Input: dimensioned drawing with shaded views. Units: mm. Origin: part minimum x, y, z. A direction names the side the tool comes from. Give positions to 0.01 mm unless a question says otherwise; leave off trailing zeros. Loops run counter-clockwise (first coordinate to the right, second up) from the corner with the lowest first, then second, coordinate; pieces in that order, holes last. Notation, with made-up numbers: (65, 57) -> (73, 57) arc R4 cw to (73, 62) -> close; hole circle Ø8 at (82.5, -27). An arc over 180 degrees is marked (long way). One line per question, with ' | ' between items. Start each with the question number.
Item 1: Section A-A on z = 42.5. Return loops of the section in (x, y).
Item 2: Set-up query: the marked faces 4 and 5. Return all of +Z, -Z, +X, -X, +Y, -Y with unobstructed straight access to the full face (end or side cutting, diameter ignored); none if empty.
Item 3: Mould query, pull axis Z, two halves, no side actions, for the marked faces 1, 2 and 3. Classes: released by +Z, released by -Z, zero draft, split by the parting line, or undercut.
Item 4: Section C-C on y = 18.75. Return loops of the section in (x, z).
Item 5: Pin query (flat end, axial travel): P1, Ø1, axis at x = 8.5, y = 8, coming from the +Z side (1 decimal); P2, Ø5, axis at x = 19.5, z = 11.5, coming from the +Y side; P3, Ø1.9, axis at x = 22.5, y = 12.5, coming from the +Z side. Return the tip coordinate at first contact, or that it passes through.
Item 6: Material intervals for line 1 along Y through (x, z) = (8, 7.5); line 2 along Y through (x, z) = (30, 16); line 3 along Y through (x, z) = (12, 35.5), sorted ascending. Write a range as [from, to].
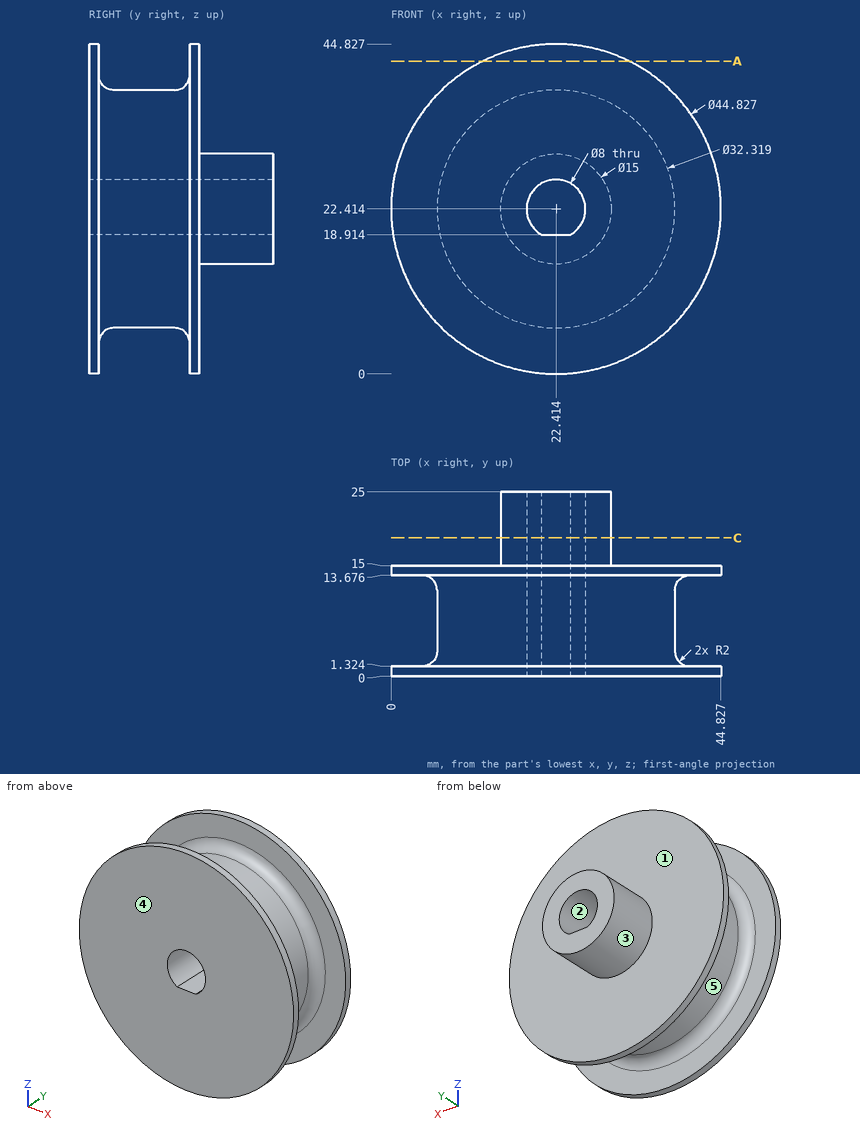
Result sheet:
1) outline: (12.47, 0) -> (32.36, 0) -> (32.36, 1.32) -> (12.47, 1.32) -> close; (12.47, 13.68) -> (32.36, 13.68) -> (32.36, 15) -> (12.47, 15) -> close
2) face 4: +Z, -Z, +X, -X, -Y | face 5: none
3) face 1: zero draft | face 2: undercut | face 3: split by the parting line
4) outline: circle Ø15 at (22.41, 22.41); hole (20.48, 18.91) -> (24.35, 18.91) arc R4 ccw (long way) to start
5) P1: stops at z = 31.4 | P2: stops at y = 15 | P3: stops at z = 39.65
6) line 1: y = [0, 1.32], [13.68, 15] | line 2: y = [0, 15] | line 3: y = [0, 1.93], [13.07, 15]
